Source: CAD feature listing. Evaluate the final solid. Frame: model axes, mm. Round coordinates to 2 decimals unless told otherwise and drop trailing zeros. Write each loop counter-clockwise with the first axis right and the second up, starting at its lowest first coordinate (ties: lowest second). Pieces come first, ordered by that corner, then holes. Notation, with made-up numbers: M 36.5,66.25 L 58.5,66.25 A16 ccw 58.5,93.25 Z; hole C 10.25,65 d11. An arc over 180 degrees is marked long. Answer in a Markdown table with one row per item. Add a question column.
Item 1: Contact query for flat-ended pins moving along their axis: pin 1 (1.8 mm diameter, centred on x = -60.65, z = -77.31, fed in from -Y); pin 2 (2.5 mm diameter, centred on x = 11.5, z = -34.18, fed in from -Y); pin 3 (1.8 mm diameter, centred on y = 4.5, z = 89.5, fed in from -X). Output: stop coordinate, or through.
Item 2: Cut plane A-A on x = -5. Return loops of the section in (y, z).
Item 3: Cut plane B-B on y = 1.05. Give the number of separate pieces and of enclosed holes in the cut face, and give its area (3 significant figures).
Item 4: Material intervals for probe 1 along X at (y, z) = (1.8, -67); probe 2 along Z at (x, y) = (26.5, 1); probe 3 along Z at (x, y) = (18.5, 1.3), sorted ascending.
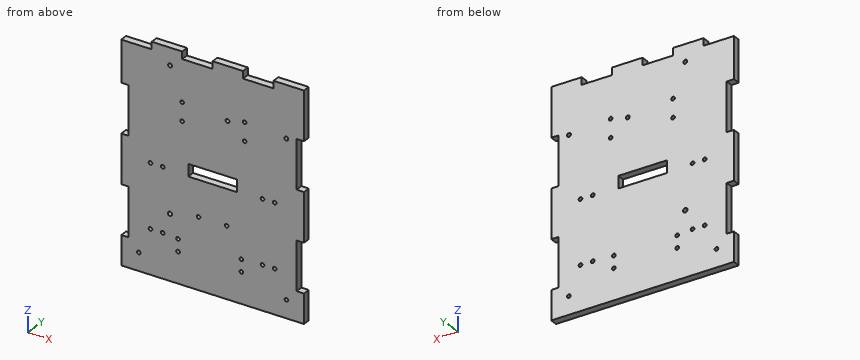
from build123d import *

# Parameters (mm, degrees)
SKETCH1_W                = 150
SKETCH1_H                = 184
BOSS_EXTRUDE1_DEPTH      = 6
SKETCH2_W                = 6
SKETCH2_H                = 40
CUT_EXTRUDE1_DEPTH       = 6
SKETCH11_W               = 25
SKETCH11_H               = 6
CUT_EXTRUDE10_DEPTH      = 6
CUT_EXTRUDE11_REACH      = 120.849
SKETCH12_R               = 1.6
CUT_EXTRUDE12_REACH      = 120.849
SKETCH13_R               = 1.8
CUT_EXTRUDE13_REACH      = 120.849
SKETCH14_R               = 1.6
CUT_EXTRUDE14_REACH      = 120.849
SKETCH15_W               = 40
SKETCH15_H               = 10
SKETCH16_R               = 1.5
CUT_EXTRUDE15_DEPTH      = 6
SKETCH17_R               = 1.5
CUT_EXTRUDE16_DEPTH      = 6
CUT_EXTRUDE17_DEPTH      = 119.966381806
CUT_EXTRUDE17_DEPTH_BACK = 7.5
SKETCH18_R               = 1.5


with BuildPart() as part:
    # Sketch1 → Boss-Extrude1 (new body)
    with BuildSketch(Plane(origin=(0, 0, 0), x_dir=(1, 0, 0), z_dir=(0, 1, 0))):
        Rectangle(SKETCH1_W, SKETCH1_H)
    extrude(amount=BOSS_EXTRUDE1_DEPTH)

    # Sketch2 → Cut-Extrude1 (cut)
    with BuildSketch(Plane(origin=(0, 6, 0), x_dir=(1, 0, 0), z_dir=(0, 1, 0))):
        with Locations((-72, 48)):
            Rectangle(SKETCH2_W, SKETCH2_H)
        with Locations((72, 48)):
            Rectangle(SKETCH2_W, SKETCH2_H)
        with Locations((72, -32)):
            Rectangle(SKETCH2_W, SKETCH2_H)
        with Locations((-72, -32)):
            Rectangle(SKETCH2_W, SKETCH2_H)
    extrude(amount=-CUT_EXTRUDE1_DEPTH, mode=Mode.SUBTRACT)

    # Sketch11 → Cut-Extrude10 (cut)
    with BuildSketch(Plane(origin=(0, 6, 0), x_dir=(1, 0, 0), z_dir=(0, 1, 0))):
        with Locations((-12.5, -89)):
            Rectangle(SKETCH11_W, SKETCH11_H)
        with Locations((-62.5, -89)):
            Rectangle(SKETCH11_W, SKETCH11_H)
        with Locations((37.5, -89)):
            Rectangle(SKETCH11_W, SKETCH11_H)
    extrude(amount=-CUT_EXTRUDE10_DEPTH, mode=Mode.SUBTRACT)

    # Sketch12 → Cut-Extrude11 (cut, up to next)
    with BuildSketch(Plane(origin=(0, 6, 0), x_dir=(1, 0, 0), z_dir=(0, 1, 0)), mode=Mode.PRIVATE) as cut_extrude11_sk1:
        with Locations(Location((-35, -78, 0), (0, 0, 270))):
            Circle(SKETCH12_R)
    cut_extrude11_tool1 = extrude(cut_extrude11_sk1.sketch, amount=-CUT_EXTRUDE11_REACH, mode=Mode.PRIVATE) & part.part
    add(cut_extrude11_tool1.solids().sort_by_distance((-35, 6, 78))[0], mode=Mode.SUBTRACT)

    # Sketch13 → Cut-Extrude12 (cut, up to next)
    with BuildSketch(Plane(origin=(0, 6, 0), x_dir=(1, 0, 0), z_dir=(0, 1, 0)), mode=Mode.PRIVATE) as cut_extrude12_sk1:
        with Locations(Location((-35, 39, 0), (0, 0, 270))):
            Circle(SKETCH13_R)
    cut_extrude12_tool1 = extrude(cut_extrude12_sk1.sketch, amount=-CUT_EXTRUDE12_REACH, mode=Mode.PRIVATE) & part.part
    add(cut_extrude12_tool1.solids().sort_by_distance((-35, 6, -39))[0], mode=Mode.SUBTRACT)

    # Sketch14 → Cut-Extrude13 (cut, up to next)
    with BuildSketch(Plane(origin=(0, 6, 0), x_dir=(1, 0, 0), z_dir=(0, 1, 0)), mode=Mode.PRIVATE) as cut_extrude13_sk1:
        with Locations(Location((12.25, -48.7, 0), (0, 0, 270))):
            Circle(SKETCH14_R)
    cut_extrude13_tool1 = extrude(cut_extrude13_sk1.sketch, amount=-CUT_EXTRUDE13_REACH, mode=Mode.PRIVATE) & part.part
    # Sketch14 → Cut-Extrude13 (cut, up to next)
    with BuildSketch(Plane(origin=(0, 6, 0), x_dir=(1, 0, 0), z_dir=(0, 1, 0)), mode=Mode.PRIVATE) as cut_extrude13_sk2:
        with Locations(Location((60.5, -49.7, 0), (0, 0, 270))):
            Circle(SKETCH14_R)
    cut_extrude13_tool2 = extrude(cut_extrude13_sk2.sketch, amount=-CUT_EXTRUDE13_REACH, mode=Mode.PRIVATE) & part.part
    add(cut_extrude13_tool1.solids().sort_by_distance((12.25, 6, 48.7))[0], mode=Mode.SUBTRACT)
    add(cut_extrude13_tool2.solids().sort_by_distance((60.5, 6, 49.7))[0], mode=Mode.SUBTRACT)

    # Sketch15 → Cut-Extrude14 (cut, up to next)
    with BuildSketch(Plane(origin=(0, 6, 0), x_dir=(1, 0, 0), z_dir=(0, 1, 0)), mode=Mode.PRIVATE) as cut_extrude14_sk1:
        Rectangle(SKETCH15_W, SKETCH15_H)
    cut_extrude14_tool1 = extrude(cut_extrude14_sk1.sketch, amount=-CUT_EXTRUDE14_REACH, mode=Mode.PRIVATE) & part.part
    add(cut_extrude14_tool1.solids().sort_by_distance((0, 6, 0))[0], mode=Mode.SUBTRACT)

    # Sketch16 → Cut-Extrude15 (cut)
    with BuildSketch(Plane.XZ):
        with Locations(Location((60.647463996, -77.306917024, 0), (0, 0, 270))):
            Circle(SKETCH16_R)
        with Locations(Location((50.984493528, -55.803329236, 0), (0, 0, 270))):
            Circle(SKETCH16_R)
        with Locations(Location((40.984493528, -55.803329236, 0), (0, 0, 270))):
            Circle(SKETCH16_R)
        with Locations(Location((50.984493528, -3.803329236, 0), (0, 0, 270))):
            Circle(SKETCH16_R)
        with Locations(Location((40.984493528, -3.803329236, 0), (0, 0, 270))):
            Circle(SKETCH16_R)
        with Locations(Location((26.276108361, 37, 0), (0, 0, 270))):
            Circle(SKETCH16_R)
        with Locations(Location((26.276108361, 52, 0), (0, 0, 270))):
            Circle(SKETCH16_R)
        with Locations(Location((-25, 52, 0), (0, 0, 270))):
            Circle(SKETCH16_R)
        with Locations(Location((-25, 37, 0), (0, 0, 270))):
            Circle(SKETCH16_R)
        with Locations(Location((-40.984493528, -3.803329236, 0), (0, 0, 270))):
            Circle(SKETCH16_R)
        with Locations(Location((-50.984493528, -3.803329236, 0), (0, 0, 270))):
            Circle(SKETCH16_R)
        with Locations(Location((-40.984493528, -55.803329236, 0), (0, 0, 270))):
            Circle(SKETCH16_R)
        with Locations(Location((-50.984493528, -55.803329236, 0), (0, 0, 270))):
            Circle(SKETCH16_R)
        with Locations(Location((-60.647463996, -77.306917024, 0), (0, 0, 270))):
            Circle(SKETCH16_R)
    extrude(amount=-CUT_EXTRUDE15_DEPTH, mode=Mode.SUBTRACT)

    # Sketch17 → Cut-Extrude16 (cut)
    with BuildSketch(Plane(origin=(0, 6, 0), x_dir=(1, 0, 0), z_dir=(0, 1, 0))):
        with Locations(Location((-28.38838906, 66.73080713, 0), (0, 0, 270))):
            Circle(SKETCH17_R)
        with Locations(Location((-28.38838906, 56.73080713, 0), (0, 0, 270))):
            Circle(SKETCH17_R)
        with Locations(Location((23.61161094, 56.73080713, 0), (0, 0, 270))):
            Circle(SKETCH17_R)
        with Locations(Location((23.61161094, 66.73080713, 0), (0, 0, 270))):
            Circle(SKETCH17_R)
    extrude(amount=-CUT_EXTRUDE16_DEPTH, mode=Mode.SUBTRACT)

    # Sketch18 → Cut-Extrude17 (cut, two sides: drawn at the far end of the back side and taken through both)
    with BuildSketch(Plane(origin=(0, -2, 0), x_dir=(-1, 0, 0), z_dir=(0, -1, 0)).offset(-CUT_EXTRUDE17_DEPTH_BACK)):
        with Locations(Location((11.5, 34.184592899, 0), (0, 0, 90))):
            Circle(SKETCH18_R)
        with Locations(Location((-11.5, 34.184592899, 0), (0, 0, 90))):
            Circle(SKETCH18_R)
    extrude(amount=CUT_EXTRUDE17_DEPTH + CUT_EXTRUDE17_DEPTH_BACK, mode=Mode.SUBTRACT)


solid = part.part
Results below:
| question | item | result |
|---|---|---|
| 1 | pin 1 | through |
| 1 | pin 2 | y = 5.5 |
| 1 | pin 3 | x = -50 |
| 2 | outline | M 0,-92 L 6,-92 L 6,-5 L 0,-5 Z; M 0,5 L 6,5 L 6,86 L 0,86 Z |
| 3 | separate pieces | 1 |
| 3 | enclosed holes | 25 |
| 3 | area | 25,600 mm2 |
| 4 | probe 1 | -69 to -29.86, -26.91 to 22.14, 25.09 to 69 |
| 4 | probe 2 | -92 to 35.52, 38.48 to 50.52, 53.48 to 86 |
| 4 | probe 3 | -92 to -5, 5 to 92 |
